from build123d import *

# Parameters (mm, degrees)
BRIDA_START           = -2
BRIDA_BASE1_OUTLINE_R = 4
BRIDA_BASE1_DEPTH     = 2
CROQUIS6_R            = 2
CROQUIS6_R_2          = 11
CORTAR_EXTRUIR1_DEPTH = 10


# Read off the part's stored shape, not the designer's step: Brida base1
with BuildPart() as part:
    # Brida base1 outline → Brida base1 (new body)
    with BuildSketch(Plane(origin=(0, 0, 0), x_dir=(1, 0, 0), z_dir=(0, 1, 0)).offset(BRIDA_START)):
        Polygon((5, 35), (5, 0), (30, 0), (30, 130), (-30, 130), (-30, 0), (-5, 0), (-5, 35), (-2.5, 35), (-2.5, 10), (2.5, 10), (2.5, 35), align=None)
        with BuildLine():
            ThreePointArc((-24, 10), (-23.18981381, 18.404759548), (-20.789091679, 26.5))
            ThreePointArc((-20.789091679, 26.5), (-15.580992435, 28.708099244), (-13.372893192, 23.5))
            ThreePointArc((-13.372893192, 23.5), (-15.33712039, 16.876621448), (-16, 10))
            ThreePointArc((-16, 10), (-20, 6), (-24, 10))
        make_face(mode=Mode.SUBTRACT)
        with Locations((20, 10)):
            Circle(BRIDA_BASE1_OUTLINE_R, mode=Mode.SUBTRACT)
    extrude(amount=BRIDA_BASE1_DEPTH)

    # Croquis6 → Cortar-Extruir1 (cut)
    with BuildSketch(Plane(origin=(0, 0, 0), x_dir=(1, 0, 0), z_dir=(0, 1, 0))):
        with Locations(Location((25, 123.945, 0), (0, 0, 270))):
            Circle(CROQUIS6_R)
        with Locations(Location((25, 95.945, 0), (0, 0, 270))):
            Circle(CROQUIS6_R)
        with Locations(Location((-15, 123.945, 0), (0, 0, 270))):
            Circle(CROQUIS6_R)
        with Locations(Location((-15, 95.945, 0), (0, 0, 270))):
            Circle(CROQUIS6_R)
        with Locations(Location((-3.845, 109.945, 0), (0, 0, 270))):
            Circle(CROQUIS6_R_2)
    extrude(amount=-CORTAR_EXTRUIR1_DEPTH, mode=Mode.SUBTRACT)


solid = part.part
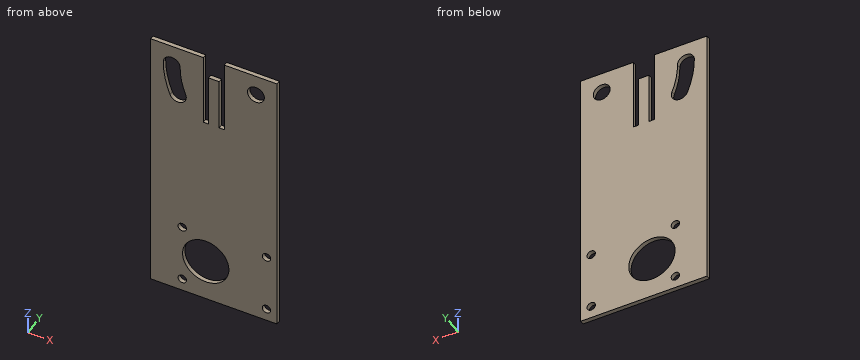
The listing builds one solid part. Answer for the finished solid, in the listing's coordinates (mm). Coordinates: 2 decimals unless noted, no trailing zeros. Loops run counter-clockwise (first coordinate to the right, second up) from the corner with the lowest first, then second, coordinate; pieces in that order, holes last.
1) A flat-ended cylindrical pin translates along its axis: pin 1 Ø2.5 at (x, z) = (25, -95.945) entering from +Y. Find the tip coordinate at first contact, or state that the pin passes through.
2) Find the intervals of material crossed by L1, parallel to Z at x = 20, y = -1.3; L2, parallel to X at y = -0.05, z = -25; L3, parallel to X at y = -1.55, z = -123.5, in increasing order.
3) Find section A-A on z = -109.5. Write down the section's boundary in (x, y), then the cut area to 3 significant figures.
4) Find section D-D on x = -18.5. Write down the section's boundary in (y, z), then the cut area to 3 significant figures.
5) Find section C-C on y = -0.9. Write down the section's boundary in (x, z) (3 decimals).
6) Find section B-B on z = -25. Write down the section's boundary in (x, y), then the cut area to 3 significant figures.
Values:
1. pin 1: passes through
2. L1: z = -130 to -14, -6 to 0
2. L2: x = -30 to -21.36, -13.08 to -5, -2.5 to 2.5, 5 to 30
2. L3: x = -30 to -16.95, -13.05 to 23.05, 26.95 to 30
3. outline: (-30, -2) - (-14.84, -2) - (-14.84, 0) - (-30, 0) - close; (7.15, -2) - (30, -2) - (30, 0) - (7.15, 0) - close
3. area: 76.0 mm2
4. outline: (-2, -130) - (0, -130) - (0, -28.74) - (-2, -28.74) - close; (-2, -6.29) - (0, -6.29) - (0, 0) - (-2, 0) - close
4. area: 215 mm2
5. outline: (-30, -130) - (30, -130) - (30, 0) - (5, 0) - (5, -35) - (2.5, -35) - (2.5, -10) - (-2.5, -10) - (-2.5, -35) - (-5, -35) - (-5, 0) - (-30, 0) - close; hole (-24, -10) arc R44 ccw to (-20.789, -26.5) arc R4 ccw to (-13.373, -23.5) arc R36 cw to (-16, -10) arc R4 ccw to start; hole circle Ø4 at (-15, -123.945); hole circle Ø4 at (-15, -95.945); hole circle Ø22 at (-3.845, -109.945); hole circle Ø8 at (20, -10); hole circle Ø4 at (25, -123.945); hole circle Ø4 at (25, -95.945)
6. outline: (-30, -2) - (-21.36, -2) - (-21.36, 0) - (-30, 0) - close; (-13.08, -2) - (-5, -2) - (-5, 0) - (-13.08, 0) - close; (-2.5, -2) - (2.5, -2) - (2.5, 0) - (-2.5, 0) - close; (5, -2) - (30, -2) - (30, 0) - (5, 0) - close
6. area: 93.4 mm2
